from build123d import *

# Parameters (mm, degrees)
SKETCH6_W          = 300
SKETCH6_H          = 100
SKETCH6_W_2        = 277
SKETCH6_H_2        = 190
CUT_EXTRUDE1_DEPTH = 50
SHELL1_T           = -15
SKETCH7_R          = 45
CUT_EXTRUDE2_DEPTH = 50


with BuildPart() as part:
    # Sketch4 → Loft1 section 0
    with BuildSketch(Plane(origin=(0, -21.618180384, 205.683247011), x_dir=(1, 0, 0), z_dir=(0, 0.10452846326765355, -0.9945218953682733))):
        with BuildLine():
            Line((0, 2924.401999756), (-400, 2924.401999756))
            Line((-400, 2924.401999756), (-400, 3954.401999756))
            Line((-400, 3954.401999756), (0, 3954.401999756))
            Line((0, 3954.401999756), (0, 2924.401999756))
        make_face()
    # Sketch2 → Loft1 section 1
    with BuildSketch(Plane.XY):
        with BuildLine():
            Line((0, -2930), (-400, -2930))
            Line((-400, -2930), (-400, -4030))
            Line((-400, -4030), (0, -4030))
            Line((0, -4030), (0, -2930))
        make_face()
    loft()

    # Sketch6 → Cut-Extrude1 (cut)
    with BuildSketch(Plane(origin=(0, -21.618180384, 205.683247011), x_dir=(-1, 0, 0), z_dir=(0, 0.1045284632676537, -0.9945218953682733))):
        with Locations((200, -3804.401999756)):
            Rectangle(SKETCH6_W, SKETCH6_H)
        with Locations((200, -3449.401999756)):
            Rectangle(SKETCH6_W_2, SKETCH6_H_2)
    extrude(amount=-CUT_EXTRUDE1_DEPTH, mode=Mode.SUBTRACT)

    # Shell1
    shell1_openings = [part.faces().sort_by_distance(p)[0] for p in [
        (-200, -3480, 0),
        (-200, -3857.518574274, -172.348423455),
        (-350, -3807.792479506, -167.122000291),
        (-200, -3758.066384737, -161.895577128),
        (-50, -3807.792479506, -167.122000291),
        (-61.5, -3454.73720665, -130.014395831),
        (-200, -3549.21678671, -139.944599842),
        (-338.5, -3454.73720665, -130.014395831),
        (-200, -3360.25762659, -120.084191821),
        (-200, -3810.405691087, -142.258952907),
        (-200, -3457.350418232, -105.151348447),
    ]]
    offset(amount=SHELL1_T, openings=shell1_openings, kind=Kind.INTERSECTION)

    # Sketch7 → Cut-Extrude2 (cut)
    with BuildSketch(Plane(origin=(0, -3557.931546215, -1295.988905699), x_dir=(1, 0, 0), z_dir=(0, -0.9396070592858665, -0.34225513018823583))):
        with Locations(Location((-200, 1268.782237568, 0), (0, 0, 270))):
            Circle(SKETCH7_R)
    extrude(amount=-CUT_EXTRUDE2_DEPTH, mode=Mode.SUBTRACT)


solid = part.part
Work out the finished part from the listing and answer in its coordinate system (mm). A direction names the side the tool comes from. Coordinates: 2 decimals unless noted, no trailing zeros. Write each loop counter-clockwise with the first axis right and the second up, starting at its lowest first coordinate (ties: lowest second). Pieces come first, ordered by that corner, then holes. Notation, with made-up numbers: M 37,63 L 89,63 A27 ccw 89,84 Z; hole C -14.5,-24 d11. An arc over 180 degrees is marked long. Use one line per item in the form item = value. Start each with the question number.
1. A tool of negligible diameter and unlimited length cuts with its end or side. For faces 4 (the face through (-61.5, -3454, -148)), 5 (the face through (-247.2, -3992.7, -102.4)), 6 (the face through (-158.85, -3325.63, -126.5)), from which of +Z, -Z, +X, -X, +Y, -Y can it reach the whole face along a straight path? Write none if from no direction.
2. Each of these flat-tipped pins is pushed along its axis until it touches: P1, Ø4, axis at x = -110, z = -147, coming from the +Y side; P2, Ø12, axis at x = -193, z = -152, coming from the +Y side; P3, Ø5, axis at y = -3063, z = -52.5, coming from the +X side; P4, Ø10, axis at x = -129.5, y = -3283.5, coming from the -Z side. Where does it stop, or does it pass through?
3. The mould has two halves that part along Y. Classify faces 1 (the face through (-50, -3807, -185)), 2 (the face through (-157.62, -3319.31, -140.92)), 3 (the face through (-387, -3501, 0)): released by +Y, released by -Y, zero draft, split by the parting line, or undercut.
4. The part is cut by section A-A (x = -271). Give the vertices of the cut face in (y, z).
5. Straight lines are drawn through the part: probe 1 along X at (y, z) = (-3829.5, -47); probe 2 along Y at (x, z) = (-167.5, -48); probe 3 along Y at (x, z) = (-50, -73). For each, find the intervals that lie inside material, in ascending order. Write a range as from..to.
6. The part is cut by section B-B (x = -38). Give the vertices of the cut face in (y, z), plus the area to 3 significant figures.
Evaluation:
q1.face_4 = +Z, -Z
q1.face_5 = -Z, +X, -X, -Y
q1.face_6 = +Z
q2.P1 = -3959.76
q2.P2 = -3547.32
q2.P3 = 0
q2.P4 = -137.68
q3.face_1 = undercut
q3.face_2 = released by +Y
q3.face_3 = zero draft
q4.outline = M -4030,0 L -3954.36,-207.66 L -3854.91,-197.21 L -3856.47,-182.29 L -3944.27,-191.52 L -4014.04,0 Z; M -3757.02,-171.84 L -3755.45,-186.76 L -3546.6,-164.81 L -3548.17,-149.89 Z; M -3359.21,-130.03 L -3357.64,-144.95 L -2930,-100 L -2930,0 L -2945,0 L -2945,-86.49 Z
q5.probe_1 = -400..-385, -15..0
q5.probe_2 = -4012.52..-3996.55, -2945..-2930
q5.probe_3 = -4003.41..-3987.45, -2945..-2930
q6.outline = M -4030,0 L -3954.36,-207.66 L -2930,-100 L -2930,0 L -2945,0 L -2945,-86.49 L -3944.27,-191.52 L -4014.04,0 Z
q6.area = 19,800 mm^2
